Geometry check sheet. Reference: the model listing, model coordinates, mm. A direction names the side the tool comes from. Give positions to 0.01 mm unless a question says otherwise; leave off trailing zeros. Write each loop counter-clockwise with the first axis right and the second up, starting at its lowest first coordinate (ties: lowest second). Pieces come first, ordered by that corner, then holes. Notation, with made-up numbers: M -6,36.25 L 21,36.25 A32 cw 21,63.25 Z; hole C 32.25,-20.75 d11. An arc over 180 degrees is marked long. Use one line per item in the form item = value. Start each with the question number.
```python
from build123d import *

# Parameters (mm, degrees)
CYLINDER1831_R               = 1.5
CYLINDER1831_DEPTH           = 50
CYLINDER1831_ROLL_ANGLE      = -22.499828
CYLINDER1831_PITCH_ANGLE     = 89.998999
CYLINDER1831_PLACEMENT_ANGLE = 22.499828
CYLINDER1835_R               = 3
CYLINDER1835_DEPTH           = 10
CYLINDER1835_PITCH_ANGLE     = 90
CYLINDER1835_PLACEMENT_ANGLE = 45
CYLINDER1832_R               = 20
CYLINDER1832_DEPTH           = 7
BOX735_W                     = 1.4
BOX735_H                     = 60
BOX735_DEPTH                 = 7
BOX735_PLACEMENT_ANGLE       = 5.7
BOX734_W                     = 1.4
BOX734_H                     = 60
BOX734_DEPTH                 = 7
BOX734_PLACEMENT_ANGLE       = 3
CUT548_PLACEMENT_ANGLE       = 134.9
BOX738_W                     = 60
BOX738_H                     = 60
BOX738_DEPTH                 = 7
BOX738_PLACEMENT_ANGLE       = 1
BOX733_W                     = 60
BOX733_H                     = 60
BOX733_DEPTH                 = 7
BOX733_PLACEMENT_ANGLE       = 2
BOX739_W                     = 120
BOX739_H                     = 60
BOX739_DEPTH                 = 7
TUBE094_R                    = 21.4
TUBE094_R_2                  = 20
TUBE094_DEPTH                = 7
BOX732_W                     = 60
BOX732_H                     = 60
BOX732_DEPTH                 = 7
BOX732_PLACEMENT_ANGLE       = 20
BOX731_W                     = 60
BOX731_H                     = 60
BOX731_DEPTH                 = 7
BOX731_PLACEMENT_ANGLE       = 20
BOX737_W                     = 120
BOX737_H                     = 60
BOX737_DEPTH                 = 7
TUBE093_R                    = 21.4
TUBE093_R_2                  = 20
TUBE093_DEPTH                = 7
CUT552_PLACEMENT_ANGLE       = 135
CYLINDER1834_R               = 1.5
CYLINDER1834_DEPTH           = 20
CYLINDER1834_PLACEMENT_ANGLE = 135
CYLINDER1833_R               = 1.5
CYLINDER1833_DEPTH           = 20
CYLINDER1833_PLACEMENT_ANGLE = 45
BOX736_W                     = 30.2
BOX736_H                     = 30.2
BOX736_DEPTH                 = 100
BOX736_PLACEMENT_ANGLE       = 45
CYLINDER1836_R               = 24
CYLINDER1836_DEPTH           = 7


with BuildPart() as obj1:
    # Cylinder1831 → Cylinder1831 (new body)
    with BuildSketch(Plane.XY):
        Circle(CYLINDER1831_R)
    extrude(amount=CYLINDER1831_DEPTH)


with BuildPart() as obj1_1:
    # Cylinder1831 roll: moved
    add(obj1.part.rotate(Axis((0, 0, 0), (1, 0, 0)), CYLINDER1831_ROLL_ANGLE))


with BuildPart() as obj1_2:
    # Cylinder1831 pitch: moved
    add(obj1_1.part.rotate(Axis((0, 0, 0), (0, 1, 0)), CYLINDER1831_PITCH_ANGLE))


with BuildPart() as obj1_3:
    # Cylinder1831 placement: moved
    add(obj1_2.part.moved(Location((0, 0, -18.5))).rotate(Axis((0, 0, -18.5), (0, 0, 1)), CYLINDER1831_PLACEMENT_ANGLE))


with BuildPart() as obj2:
    # Cylinder1835 → Cylinder1835 (new body)
    with BuildSketch(Plane.XY):
        Circle(CYLINDER1835_R)
    extrude(amount=CYLINDER1835_DEPTH)


with BuildPart() as obj2_1:
    # Cylinder1835 pitch: moved
    add(obj2.part.rotate(Axis((0, 0, 0), (0, 1, 0)), CYLINDER1835_PITCH_ANGLE))


with BuildPart() as obj2_2:
    # Cylinder1835 placement: moved
    add(obj2_1.part.moved(Location((14.849242, 14.849242, -18.5))).rotate(Axis((14.849242, 14.849242, -18.5), (0, 0, 1)), CYLINDER1835_PLACEMENT_ANGLE))


with BuildPart() as obj3:
    # Cylinder1832 → Cylinder1832 (new body)
    with BuildSketch(Plane.XY.offset(-22)):
        Circle(CYLINDER1832_R)
    extrude(amount=CYLINDER1832_DEPTH)


with BuildPart() as krychle735:
    # Box735 → Box735 (new body)
    with BuildSketch(Plane.XY):
        with Locations((0.7, 30)):
            Rectangle(BOX735_W, BOX735_H)
    extrude(amount=BOX735_DEPTH)


with BuildPart() as krychle735_1:
    # Box735 placement: moved
    add(krychle735.part.moved(Location((0, 0, -22))).rotate(Axis((0, 0, -22), (0, 0, 1)), BOX735_PLACEMENT_ANGLE))


with BuildPart() as cut548:
    # Box734 → Box734 (new body)
    with BuildSketch(Plane.XY):
        with Locations((0.7, 30)):
            Rectangle(BOX734_W, BOX734_H)
    extrude(amount=BOX734_DEPTH)


with BuildPart() as cut548_1:
    # Box734 placement: moved
    add(cut548.part.moved(Location((0, 0, -22))).rotate(Axis((0, 0, -22), (0, 0, -1)), BOX734_PLACEMENT_ANGLE))

    # Compound905: union Krychle735
    add(krychle735_1.part)

    # Cut548: cut obj3
    add(obj3.part, mode=Mode.SUBTRACT)


with BuildPart() as cut548_2:
    # Cut548 placement: moved
    add(cut548_1.part.rotate(Axis((0, 0, 0), (0, 0, 1)), CUT548_PLACEMENT_ANGLE))


with BuildPart() as krychle738:
    # Box738 → Box738 (new body)
    with BuildSketch(Plane.XY):
        with Locations((30, 30)):
            Rectangle(BOX738_W, BOX738_H)
    extrude(amount=BOX738_DEPTH)


with BuildPart() as krychle738_1:
    # Box738 placement: moved
    add(krychle738.part.moved(Location((-59.990862, -1.047144, -22))).rotate(Axis((-59.990862, -1.047144, -22), (0, 0, 1)), BOX738_PLACEMENT_ANGLE))


with BuildPart() as compound904:
    # Box733 → Box733 (new body)
    with BuildSketch(Plane.XY):
        with Locations((30, 30)):
            Rectangle(BOX733_W, BOX733_H)
    extrude(amount=BOX733_DEPTH)


with BuildPart() as compound904_1:
    # Box733 placement: moved
    add(compound904.part.moved(Location((0, 0, -22))).rotate(Axis((0, 0, -22), (0, 0, -1)), BOX733_PLACEMENT_ANGLE))

    # Compound904: union Krychle738
    add(krychle738_1.part)


with BuildPart() as krychle739:
    # Box739 → Box739 (new body)
    with BuildSketch(Plane(origin=(-60, -60, -22), x_dir=(1, 0, 0), z_dir=(0, 0, 1))):
        with Locations((60, 30)):
            Rectangle(BOX739_W, BOX739_H)
    extrude(amount=BOX739_DEPTH)


with BuildPart() as cut554:
    # Tube094 → Tube094 (new body)
    with BuildSketch(Plane.XY.offset(-22)):
        Circle(TUBE094_R)
        Circle(TUBE094_R_2, mode=Mode.SUBTRACT)
    extrude(amount=TUBE094_DEPTH)

    # Cut555: cut Krychle739
    add(krychle739.part, mode=Mode.SUBTRACT)

    # Cut554: cut Compound904
    add(compound904_1.part, mode=Mode.SUBTRACT)


with BuildPart() as cut554_1:
    # Cut554 placement: moved
    add(cut554.part.moved(Location((0, 0, -7))))


with BuildPart() as krychle732:
    # Box732 → Box732 (new body)
    with BuildSketch(Plane.XY):
        with Locations((30, 30)):
            Rectangle(BOX732_W, BOX732_H)
    extrude(amount=BOX732_DEPTH)


with BuildPart() as krychle732_1:
    # Box732 placement: moved
    add(krychle732.part.moved(Location((-56.381557, -20.521209, -22))).rotate(Axis((-56.381557, -20.521209, -22), (0, 0, 1)), BOX732_PLACEMENT_ANGLE))


with BuildPart() as compound907:
    # Box731 → Box731 (new body)
    with BuildSketch(Plane.XY):
        with Locations((30, 30)):
            Rectangle(BOX731_W, BOX731_H)
    extrude(amount=BOX731_DEPTH)


with BuildPart() as compound907_1:
    # Box731 placement: moved
    add(compound907.part.moved(Location((0, 0, -22))).rotate(Axis((0, 0, -22), (0, 0, -1)), BOX731_PLACEMENT_ANGLE))

    # Compound907: union Krychle732
    add(krychle732_1.part)


with BuildPart() as krychle737:
    # Box737 → Box737 (new body)
    with BuildSketch(Plane(origin=(-60, -60, -22), x_dir=(1, 0, 0), z_dir=(0, 0, 1))):
        with Locations((60, 30)):
            Rectangle(BOX737_W, BOX737_H)
    extrude(amount=BOX737_DEPTH)


with BuildPart() as cut552:
    # Tube093 → Tube093 (new body)
    with BuildSketch(Plane.XY.offset(-22)):
        Circle(TUBE093_R)
        Circle(TUBE093_R_2, mode=Mode.SUBTRACT)
    extrude(amount=TUBE093_DEPTH)

    # Cut559: cut Krychle737
    add(krychle737.part, mode=Mode.SUBTRACT)

    # Cut556: cut Compound907
    add(compound907_1.part, mode=Mode.SUBTRACT)


with BuildPart() as cut552_1:
    # Cut556 placement: moved
    add(cut552.part.moved(Location((0, 0, -7))))

    # Cut552: cut Cut554
    add(cut554_1.part, mode=Mode.SUBTRACT)


with BuildPart() as cut552_2:
    # Cut552 placement: moved
    add(cut552_1.part.moved(Location((0, 0, 7))).rotate(Axis((0, 0, 7), (0, 0, 1)), CUT552_PLACEMENT_ANGLE))


with BuildPart() as obj4:
    # Cylinder1834 → Cylinder1834 (new body)
    with BuildSketch(Plane.XY):
        Circle(CYLINDER1834_R)
    extrude(amount=CYLINDER1834_DEPTH)


with BuildPart() as obj4_1:
    # Cylinder1834 placement: moved
    add(obj4.part.moved(Location((-14.142136, 14.142136, -30))).rotate(Axis((-14.142136, 14.142136, -30), (0, 0, 1)), CYLINDER1834_PLACEMENT_ANGLE))


with BuildPart() as compound906:
    # Cylinder1833 → Cylinder1833 (new body)
    with BuildSketch(Plane.XY):
        Circle(CYLINDER1833_R)
    extrude(amount=CYLINDER1833_DEPTH)


with BuildPart() as compound906_1:
    # Cylinder1833 placement: moved
    add(compound906.part.moved(Location((14.142136, -14.142136, -30))).rotate(Axis((14.142136, -14.142136, -30), (0, 0, -1)), CYLINDER1833_PLACEMENT_ANGLE))

    # Compound906: union obj4
    add(obj4_1.part)


with BuildPart() as krychle736:
    # Box736 → Box736 (new body)
    with BuildSketch(Plane.XY):
        with Locations((15.1, 15.1)):
            Rectangle(BOX736_W, BOX736_H)
    extrude(amount=BOX736_DEPTH)


with BuildPart() as krychle736_1:
    # Box736 placement: moved
    add(krychle736.part.moved(Location((0, -21.354625, -30))).rotate(Axis((0, -21.354625, -30), (0, 0, 1)), BOX736_PLACEMENT_ANGLE))


with BuildPart() as cut551:
    # Cylinder1836 → Cylinder1836 (new body)
    with BuildSketch(Plane.XY.offset(-22)):
        Circle(CYLINDER1836_R)
    extrude(amount=CYLINDER1836_DEPTH)

    # Cut553: cut Krychle736
    add(krychle736_1.part, mode=Mode.SUBTRACT)

    # Cut558: cut Compound906
    add(compound906_1.part, mode=Mode.SUBTRACT)

    # Cut557: cut Cut552
    add(cut552_2.part, mode=Mode.SUBTRACT)

    # Cut549: cut Cut548
    add(cut548_2.part, mode=Mode.SUBTRACT)

    # Cut550: cut obj2
    add(obj2_2.part, mode=Mode.SUBTRACT)

    # Cut551: cut obj1
    add(obj1_3.part, mode=Mode.SUBTRACT)


solid = cut551.part
```
(1) Sectioned sample at B-B, the plane y = 12. State how many separate pieces and enclosed holes the cut face has, plus the area to 3 significant figures.
(2) Sectioned sample at A-A, the plane x = -7. Record the boundary of the cut face in (y, z).
(3) Tool access check on faces 1 (the cylindrical face through (-16.605, -11.147, -18.549)), 2 (the flat face through (15.8, 13.9, -19.8)). Record the directions out of +Z, -Z, +X, -X, +Y, -Y that give a thin tool (end or side, any length) a straight path to the whole face; none if there is none.
(4) Draft check along Y on faces 3 (the flat face through (-8.744, -18.752, -18.549)), 4 (the flat face through (-9, 13, -15)), 5 (the cylindrical face through (-17.11, -16.83, -18.55)). Enter one of: released by +Y, released by -Y, zero draft, split by the parting line, or undercut.
(5) Thickness scan on probe 1 along X at (y, z) = (-11.5, -15.5); probe 2 along X at (y, z) = (-17, -19); probe 3 along Y at (x, z) = (-18, -18). Record the ranges inside material, lowest first. Write a range as [from, to].
(6) Sectioned sample at C-C, the plane x = 8. Record the boundary of the cut face in (y, z), plus the area to 3 significant figures.
(7) Depth check by flat-ended pin: pin 1 (1.5 mm diameter, centred on x = 11.5, y = 7.5, fed in from -Z); pin 2 (3 mm diameter, centred on y = 12.5, z = -20, fed in from -X); pin 3 (1 mm diameter, centred on x = -1, z = -18.5, fed in from +Y). Enter the tip coordinate at first touch or a pass-through.
Numbers:
q1.separate_pieces = 2
q1.enclosed_holes = 1
q1.area = 150 mm2
q2.outline = M -22.96,-22 L -14.35,-22 L -14.35,-15 L -22.96,-15 Z; M 14.35,-22 L 22.96,-22 L 22.96,-15 L 14.35,-15 Z
q3.face_1 = +Z, -Z
q3.face_2 = none
q4.face_3 = undercut
q4.face_4 = zero draft
q4.face_5 = released by -Y
q5.probe_1 = [-21.07, -18.05], [-16.36, -9.85], [9.85, 21.07]
q5.probe_2 = [-16.94, -15.78], [-13.96, -13], [-10.54, -4.35], [4.35, 16.94]
q5.probe_3 = [-14.27, -11.57], [-8.72, -3.35], [3.35, 15.87]
q6.outline = M -22.63,-22 L -13.35,-22 L -13.35,-15 L -22.63,-15 Z; M 13.35,-22 L 22.63,-22 L 22.63,-15 L 13.35,-15 Z
q6.area = 130 mm2
q7.pin_1 = through
q7.pin_2 = -21.33
q7.pin_3 = 23.99
